Work out the finished part from the listing and answer in its coordinate system (mm). A direction names the side the tool comes from. Coordinates: 2 decimals unless noted, no trailing zeros. Write each question's results on one line, items separated by ' | '. Start each with the question number.
from build123d import *

# Parameters (mm, degrees)
EXTRUDE1_DEPTH     = 12.7
SKETCH3_R          = 14.869502809
EXTRUDE2_DEPTH     = 2.54
CHAMFER1_SIZE      = 0.762
CHAMFER2_SIZE      = 0.762
SKETCH5_R          = 14.869502809
EXTRUDE3_DEPTH     = 12.7
EXTRUDE3_TAPER     = 26
SKETCH4_R          = 6.35
CUT_EXTRUDE1_DEPTH = 28.9400001
LPATTERN2_COUNT    = 17
LPATTERN2_PITCH    = 1.74


with BuildPart() as part:
    # Sketch2 → Extrude1 (new body)
    with BuildSketch(Plane.XY):
        Polygon((12.673375262, 0), (6.336687631, 10.975464929), (-6.336687631, 10.975464929), (-12.673375262, 0), (-6.336687631, -10.975464929), (6.336687631, -10.975464929), align=None)
    extrude(amount=EXTRUDE1_DEPTH)

    # Sketch3 → Extrude2 (add)
    with BuildSketch(Plane(origin=(0, 0, 0), x_dir=(-1, 0, 0), z_dir=(0, 0, -1))):
        Circle(SKETCH3_R)
    extrude(amount=EXTRUDE2_DEPTH)

    # Chamfer1
    chamfer1_edges = [part.edges().sort_by_distance(p)[0] for p in [
        (0, -10.975464929, 0),
        (-9.505031447, -5.487732464, 0),
        (-9.505031447, 5.487732464, 0),
        (0, 10.975464929, 0),
        (9.505031447, 5.487732464, 0),
        (9.505031447, -5.487732464, 0),
    ]]
    chamfer(chamfer1_edges, length=CHAMFER1_SIZE)

    # Chamfer2
    chamfer2_edges = [part.edges().sort_by_distance(p)[0] for p in [
        (0, 10.975464929, 12.7),
        (-9.505031447, 5.487732464, 12.7),
        (-9.505031447, -5.487732464, 12.7),
        (0, -10.975464929, 12.7),
        (9.505031447, -5.487732464, 12.7),
        (9.505031447, 5.487732464, 12.7),
    ]]
    chamfer(chamfer2_edges, length=CHAMFER2_SIZE)

    # Sketch5 → Extrude3 (add)
    with BuildSketch(Plane(origin=(0, 0, -2.54), x_dir=(-1, 0, 0), z_dir=(0, 0, -1))):
        Circle(SKETCH5_R)
    extrude(amount=EXTRUDE3_DEPTH, taper=EXTRUDE3_TAPER)

    # Sketch4 → Cut-Extrude1 (cut, through all)
    with BuildSketch(Plane.XY.offset(12.7)):
        Circle(SKETCH4_R)
    extrude(amount=-CUT_EXTRUDE1_DEPTH, mode=Mode.SUBTRACT)

    # Sketch7 → Cut-Revolve1 (revolve, cut)
    with BuildSketch(Plane(origin=(0, 0, 0), x_dir=(1, 0, 0), z_dir=(0, 1, 0))):
        Polygon((6.340392923, -11.96936439), (7.115488803, -12.7), (6.340392923, -13.49336439), (5.591488803, -12.7), align=None)
    cut_revolve1 = revolve(axis=Axis((0, 0, -15.24), (0, 0, 1)), mode=Mode.SUBTRACT)

    # LPattern2: Cut-Revolve1 ×17
    with Locations(*[(0, 0, -i * LPATTERN2_PITCH) for i in range(1, LPATTERN2_COUNT)]):
        add(cut_revolve1, mode=Mode.SUBTRACT)


solid = part.part
1. For faces 1 (the face through (0, 10.975, 6)), 2 (the face through (-9.215, -5.218, 12.324)), determine the directions among +Z, -Z, +X, -X, +Y, -Y from which every point of the face is accessible in a straight line to the end or side of a thin tool.
2. Find the intervals of material crossed by L1, parallel to Y at x = 0, z = -0.25; L2, parallel to Y at x = 0, z = 10.1; L3, parallel to X at y = 0, z = 5.05, in increasing order.
3. Given pin 1 Ø4 at (y, z) = (-3.5, -9.5) entering from +X; pin 2 Ø8 at (y, z) = (5, -7.5) entering from -X; pin 3 Ø3 at (y, z) = (0.5, 6.5) entering from +X, each flat-ended and moving along its own axis, determine where each tip first touches the part or whether it passes through.
Ans:
1) face 1: +Z, +X, -X, +Y | face 2: +Z, -X, -Y
2) L1: y = -14.87 to -6.35, 6.35 to 14.87 | L2: y = -10.98 to -6.35, 6.35 to 10.98 | L3: x = -12.67 to -6.38, 6.38 to 12.67
3) pin 1: stops at x = 12.07 | pin 2: stops at x = -13.83 | pin 3: stops at x = 12.67
